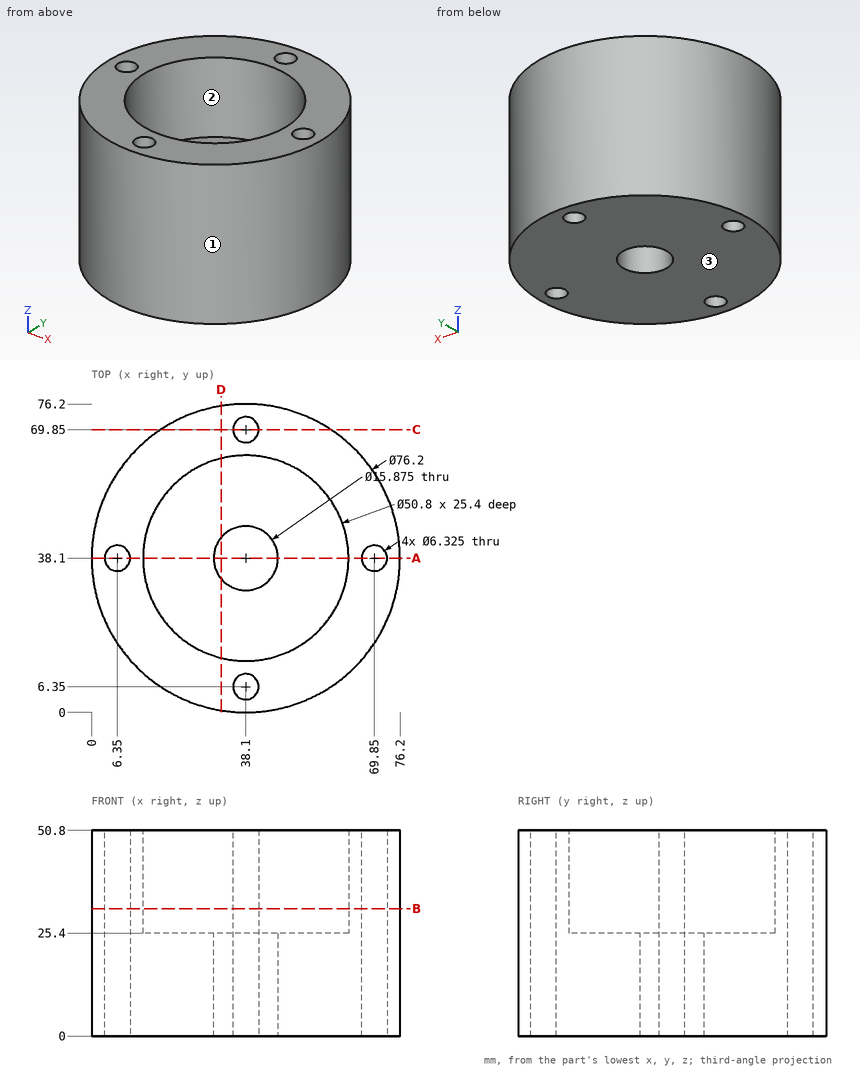
For this review, use the dimensioned drawing (mm, ordinates from the lowest corner) and the shaded views. Give positions to 0.01 mm unless a question says otherwise; leave off trailing zeros. Order: outer loops, then holes, each group sorted by start corner. A loop starts at its lowest first (then second) coordinate and runs counter-clockwise, first axis right, second up.
1) Take a section at C-C (y = 69.85). Give the boundary of the cut face in (x, z).
2) Take a section at B-B (z = 31.5). State how many separate pieces and enclosed holes the cut face has, then the cut area to 3 significant figures.
3) Insertion check: pin 1 (5 mm diameter, centred on x = 38.1, y = 6.35, fed in from +Z); pin 2 (1 mm diameter, centred on x = 40.5, y = 19.5, fed in from -Z); pin 3 (15 mm diameter, centred on x = 26.5, y = 38, fed in from +Z); pin 4 (4 mm diameter, centred on x = 44.5, z = 10, fed in from -Y) (1 decimal). Each pin has a flat end and moves straight along its axis. Give the tip position at first contact, or say it passes through.
4) Take a section at A-A (y = 38.1). Give the boundary of the cut face in (x, z).
5) Take a section at D-D (x = 32). Give the boundary of the cut face in (y, z), then the cut area to 3 significant figures.
6) The part is to be moulded in two halves that separate along Y. For the marked faces 1, 2 and 3, say which applies: released by +Y, released by -Y, zero draft, split by the parting line, or undercut.
7) Wall thickness on line 1 (Y direction, x = 38.1, z = 15.25); line 2 (Y direction, x = 41, z = 40) (1 decimal): over which ranges is each line inside the solid? List them lowest first.
Derived:
1. outline: (17.04, 0) - (34.94, 0) - (34.94, 50.8) - (17.04, 50.8) - close; (41.26, 0) - (59.16, 0) - (59.16, 50.8) - (41.26, 50.8) - close
2. separate pieces: 1
2. enclosed holes: 5
2. area: 2,410 mm2
3. pin 1: passes through
3. pin 2: stops at z = 0
3. pin 3: stops at z = 25.4
3. pin 4: stops at y = 0.3
4. outline: (0, 0) - (3.19, 0) - (3.19, 50.8) - (0, 50.8) - close; (9.51, 0) - (30.16, 0) - (30.16, 25.4) - (12.7, 25.4) - (12.7, 50.8) - (9.51, 50.8) - close; (46.04, 0) - (66.69, 0) - (66.69, 50.8) - (63.5, 50.8) - (63.5, 25.4) - (46.04, 25.4) - close; (73.01, 0) - (76.2, 0) - (76.2, 50.8) - (73.01, 50.8) - close
5. outline: (0.49, 0) - (33.02, 0) - (33.02, 25.4) - (13.44, 25.4) - (13.44, 50.8) - (0.49, 50.8) - close; (43.18, 0) - (75.71, 0) - (75.71, 50.8) - (62.76, 50.8) - (62.76, 25.4) - (43.18, 25.4) - close
5. area: 2,310 mm2
6. face 1: split by the parting line
6. face 2: undercut
6. face 3: zero draft
7. line 1: y = 0 to 3.19, 9.51 to 30.16, 46.04 to 66.69, 73.01 to 76.2
7. line 2: y = 0.1 to 5.1, 7.6 to 12.9, 63.3 to 68.6, 71.1 to 76.1
